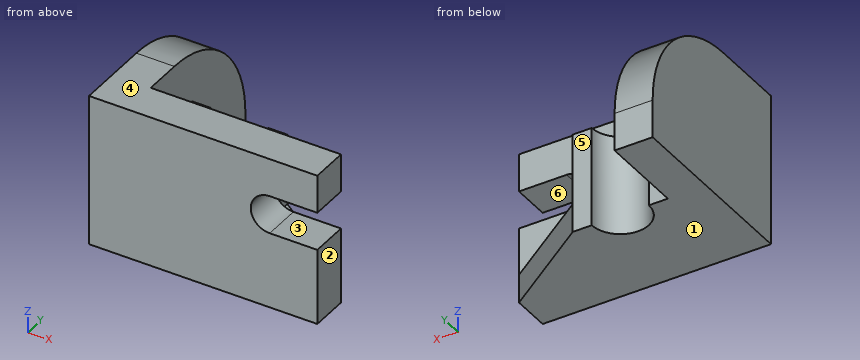
from build123d import *

# Parameters (mm, degrees)
SKETCH1_W           = 96
SKETCH1_H           = 64
BOSS_EXTRUDE1_DEPTH = 16
SKETCH2_W           = 64
SKETCH2_H           = 64
BOSS_EXTRUDE2_DEPTH = 16
FILLET2_R           = 48
SKETCH3_W           = 40
SKETCH3_H           = 42
BOSS_EXTRUDE3_DEPTH = 28
SKETCH4_R           = 12
CUT_EXTRUDE1_DEPTH  = 103.313244499
CUT_EXTRUDE2_DEPTH  = 87.162636914
BOSS_EXTRUDE5_DEPTH = 12


with BuildPart() as part:
    # Sketch1 → Boss-Extrude1 (new body)
    with BuildSketch(Plane(origin=(0, 0, 0), x_dir=(1, 0, 0), z_dir=(0, 1, 0))):
        Rectangle(SKETCH1_W, SKETCH1_H)
    extrude(amount=BOSS_EXTRUDE1_DEPTH)

    # Sketch2 → Boss-Extrude2 (add)
    with BuildSketch(Plane.ZY.offset(48)):
        with Locations((0, 48)):
            Rectangle(SKETCH2_W, SKETCH2_H)
    extrude(amount=-BOSS_EXTRUDE2_DEPTH)

    # Fillet2
    fillet2_edges = [part.edges().sort_by_distance(p)[0] for p in [
        (-40, 80, 32),
    ]]
    fillet(fillet2_edges, radius=FILLET2_R)

    # Sketch3 → Boss-Extrude3 (add)
    with BuildSketch(Plane(origin=(0, 16, 0), x_dir=(1, 0, 0), z_dir=(0, 1, 0))):
        with Locations((-12, 11)):
            Rectangle(SKETCH3_W, SKETCH3_H)
    extrude(amount=BOSS_EXTRUDE3_DEPTH)

    # Sketch4 → Cut-Extrude1 (cut, through all)
    with BuildSketch(Plane.XY.offset(10)):
        with Locations((-12, 44)):
            Circle(SKETCH4_R)
    extrude(amount=-CUT_EXTRUDE1_DEPTH, mode=Mode.SUBTRACT)

    # Sketch6 → Cut-Extrude2 (cut, through all)
    with BuildSketch(Plane(origin=(0, 16, 0), x_dir=(1, 0, 0), z_dir=(0, 1, 0))):
        with BuildLine():
            Line((48, -16), (28, -16))
            ThreePointArc((28, -16), (20, -8), (28, 0))
            Line((28, 0), (48, 0))
            ThreePointArc((48, 0), (56, -8), (48, -16))
        make_face()
    extrude(amount=-CUT_EXTRUDE2_DEPTH, mode=Mode.SUBTRACT)

    # Sketch7 → Boss-Extrude5 (add)
    with BuildSketch(Plane(origin=(0, 0, -32), x_dir=(-1, 0, 0), z_dir=(0, 0, -1))):
        Polygon((-8, 44), (-48, 16), (-8, 16), align=None)
    extrude(amount=-BOSS_EXTRUDE5_DEPTH)


solid = part.part
Design review of the part built by this model. Coordinates are the model's own, in mm. Face numbers are marked on the shaded views. A direction names the side the tool comes from. Give positions to 0.01 mm unless a question says otherwise; leave off trailing zeros. Order: outer loops, then holes, each group sorted by start corner. A loop starts at its lowest first (then second) coordinate and runs counter-clockwise, first axis right, second up. Notation, with made-up numbers: (39, -11.5) - (96, -11.5) arc R34 ccw to (96, 20.5) - close; hole circle Ø11 at (9, 68.25). An arc over 180 degrees is marked (long way). Write item = value, one per line. Start each with the question number.
Q1. Clearance check with flat-ended pins moving along their axes: pin 1 Ø15.5 at (x, z) = (25, 6) entering from +Y; pin 2 Ø1.5 at (x, y) = (-36.5, 52) entering from +Z; pin 3 Ø19 at (y, z) = (61, -6.5) entering from +X. State where each tip first meets the part, or that it passes through.
Q2. We need section A-A on x = 33. State the section outline as (y, z) points.
Q3. We need section D-D on y = 10. State the section outline as (x, z) points.
Q4. We need section B-B on z = -23. State the section outline as (x, y) points.
Q5. Tool access review of the marked faces 4, 5 and 6: name each direction out of +Z, -Z, +X, -X, +Y, -Y from which nothing blocks a thin tool from reaching the whole face with its end or side.
Q6. To check wall thickness, follow L1, parallel to X at y = 52, z = -20; L2, parallel to Y at x = 16, z = 0.5; L3, parallel to X at y = 20, z = 8.5. State the ranges of each line that lie inside material, in increasing order. Write a range as from..to.
Q7. We need section C-C on y = 37.5. State the section outline as (x, z) points.
Q8. Mouldability with a two-part tool opening along Z and no side actions: class the marked faces 1, 2 and 3 as released by +Z, released by -Z, zero draft, split by the parting line, or undercut.
Working result:
q1.pin_1 = 16
q1.pin_2 = 27.97
q1.pin_3 = -32
q2.outline = (0, -32) - (26.5, -32) - (26.5, -20) - (16, -20) - (16, 0) - (0, 0) - close; (0, 16) - (16, 16) - (16, 32) - (0, 32) - close
q3.outline = (-48, -32) - (48, -32) - (48, 0) - (28, 0) arc R8 cw to (28, 16) - (48, 16) - (48, 32) - (-48, 32) - close
q4.outline = (-48, 0) - (48, 0) - (48, 16) - (8, 44) - (0, 44) arc R12 cw to (-24, 44) - (-32, 44) - (-32, 80) - (-48, 80) - close
q5.face_4 = +Z, +X, -X, +Y, -Y
q5.face_5 = +Z, -Z, +X, +Y
q5.face_6 = +X, +Y, -Y
q6.L1 = -48..-32
q6.L2 = 0..16
q6.L3 = -48..8
q7.outline = (-48, -32) - (-22.09, -32) - (-22.09, 10) - (-32, 10) - (-32, 31.68) - (-48, 31.68) - close; (-1.91, -32) - (17.29, -32) - (17.29, -20) - (8, -20) - (8, 10) - (-1.91, 10) - close
q8.face_1 = released by -Z
q8.face_2 = zero draft
q8.face_3 = undercut
